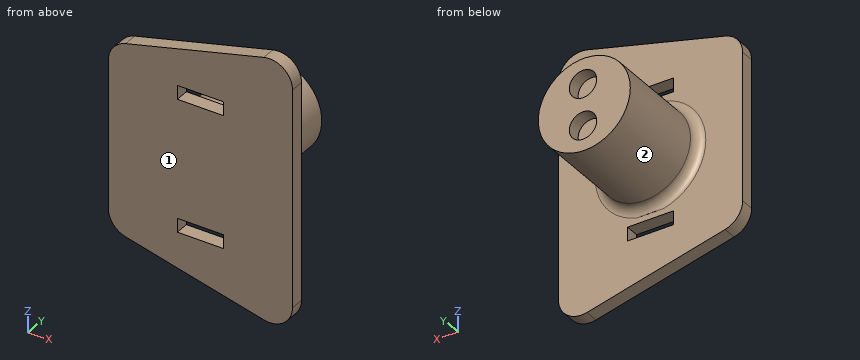
Autodesk Fusion 360 part; units mm, degrees
sketch "Sketch1" plane through (0, 0, 0) normal (0, 1, 0) x (1, 0, 0)
  line L0 (46.0121, 0.2) -> (46.0121, -59.8)
  line L1 (6.0121, -29.5532) -> (6.0121, -9.5532)
  line L2 (6.0121, -29.5532) -> (6.0121, -49.5532)
  line L3 (6.0121, -9.5532) -> (46.0121, 0.2)
  line L4 (6.0121, -49.5532) -> (46.0121, -59.8)
  line L5 (31.0121, -13.6532) -> (21.0121, -13.6532)
  line L6 (21.0121, -13.6532) -> (21.0121, -16.6532)
  line L7 (21.0121, -16.6532) -> (31.0121, -16.6532)
  line L8 (31.0121, -16.6532) -> (31.0121, -13.6532)
  line L9 (31.0121, -42.4532) -> (21.0121, -42.4532)
  line L10 (21.0121, -42.4532) -> (21.0121, -45.4532)
  line L11 (21.0121, -45.4532) -> (31.0121, -45.4532)
  line L12 (31.0121, -45.4532) -> (31.0121, -42.4532)
  point P0 (26.0121, -15.0532)
  point P1 (25.8317, -44.4989)
  dimension "d1" = 60
  dimension "d6" = 20
  dimension "d7" = 20
  dimension "d9" = 40
  dimension "d10" = 40
  dimension "d11" = 20
  dimension "d12" = 14.5
  dimension "d13" = 10
  dimension "d14" = 3
  dimension "d15" = 10
  dimension "d16" = 3
  dimension "d19" = 12.9
  dimension "d20" = 12.9
  dimension "d21" = 25.8
  dimension "d22" = 15
  dimension "d23" = 15
extrude "Extrude1" add sketch "Sketch1" along normal blind 3
sketch "Sketch2" plane through (0, 3, 0) normal (0, 1, 0) x (-1, 0, 0)
  line L0 (-31.0121, 42.4532) -> (-31.0121, 45.4532)
  line L1 (-31.0121, 45.4532) -> (-21.0121, 45.4532)
  line L2 (-21.0121, 45.4532) -> (-21.0121, 42.4532)
  line L3 (-21.0121, 42.4532) -> (-31.0121, 42.4532)
  line L4 (-31.0121, 13.6532) -> (-31.0121, 16.6532)
  line L5 (-31.0121, 16.6532) -> (-21.0121, 16.6532)
  line L6 (-21.0121, 16.6532) -> (-21.0121, 13.6532)
  line L7 (-21.0121, 13.6532) -> (-31.0121, 13.6532)
  line L8 (-6.0121, 9.5532) -> (-6.0121, 49.5532)
  line L9 (-6.0121, 49.5532) -> (-46.0121, 59.8)
  line L10 (-46.0121, 59.8) -> (-46.0121, -0.2)
  line L11 (-46.0121, -0.2) -> (-6.0121, 9.5532)
  circle A0 centre (-26.0121, 29.5532) radius 10
  point P0 (-26.0121, 29.5532)
  dimension "d38" = 12.9
  dimension "d39" = 12.9
  dimension "d42" = 20
extrude "Extrude2" add sketch "Sketch2" along normal blind 22 contours A0
sketch "Sketch3" plane through (0, 25, 0) normal (0, 1, 0) x (-1, 0, 0)
  line L0 (-28.0121, 38.7532) -> (-24.0121, 38.7532)
  line L1 (-24.0121, 38.7532) -> (-24.0121, 20.7532)
  line L2 (-24.0121, 20.7532) -> (-28.0121, 20.7532)
  line L3 (-28.0121, 20.7532) -> (-28.0121, 38.7532)
  line L4 (-28.0121, 38.7532) -> (-24.0121, 20.7532) construction
  line L5 (-24.0121, 38.7532) -> (-28.0121, 20.7532) construction
  circle A0 centre (-26.0121, 29.5532) radius 10
  point P0 (-26.0121, 29.7532)
  dimension "d28" = 18
fillet "Fillet4" radius 2 1 edges at (35.3354, 3, 33.1694)
fillet "Fillet3" radius 5 4 edges at (6.0121, 1.5, 9.5532) (6.0121, 1.5, 49.5532) (46.0121, 1.5, 59.8) (46.0121, 1.5, -0.2)
sketch "Sketch5" plane through (0, 25, 0) normal (0, 1, 0) x (-1, 0, 0)
  circle A0 centre (-26.0121, 29.5532) radius 10
  circle A1 centre (-26.282, 34.0532) radius 2.975
  circle A2 centre (-26.282, 25.0532) radius 2.975
  dimension "d48" = 5.95
  dimension "d49" = 5.95
  dimension "d50" = 4.5
  dimension "d51" = 4.5
extrude "Extrude5" cut sketch "Sketch5" against normal blind 2.93 contours A1 | A2
sketch "Sketch6" plane through (0, 3, 0) normal (0, 1, 0) x (-1, 0, 0)
  arc A0 (-46.0121, 6.1656) -> (-39.8276, 1.308) centre (-41.0121, 6.1656) ccw
  line L0 (-39.8276, 1.308) -> (-9.8276, 8.6229)
  arc A1 (-9.8276, 8.6229) -> (-6.0121, 13.4806) centre (-11.0121, 13.4806) ccw
  line L1 (-6.0121, 13.4806) -> (-6.0121, 45.6726)
  arc A2 (-6.0121, 45.6726) -> (-9.7713, 50.5162) centre (-11.0121, 45.6726) ccw
  line L2 (-9.7713, 50.5162) -> (-39.7713, 58.2013)
  arc A3 (-39.7713, 58.2013) -> (-46.0121, 53.3577) centre (-41.0121, 53.3577) ccw
  line L3 (-46.0121, 53.3577) -> (-46.0121, 6.1656)
  line L4 (-31.0121, 42.4532) -> (-31.0121, 45.4532)
  line L5 (-31.0121, 45.4532) -> (-21.0121, 45.4532)
  line L6 (-21.0121, 45.4532) -> (-21.0121, 42.4532)
  line L7 (-21.0121, 42.4532) -> (-31.0121, 42.4532)
  line L8 (-31.0121, 13.6532) -> (-31.0121, 16.6532)
  line L9 (-31.0121, 16.6532) -> (-21.0121, 16.6532)
  line L10 (-21.0121, 16.6532) -> (-21.0121, 13.6532)
  line L11 (-21.0121, 13.6532) -> (-31.0121, 13.6532)
  circle A4 centre (-26.0121, 29.5532) radius 12
  line L12 (-21.0121, 17.9232) -> (-31.0121, 17.9232)
  line L13 (-31.0121, 17.9232) -> (-31.0121, 12.3832)
  line L14 (-31.0121, 12.3832) -> (-21.0121, 12.3832)
  line L15 (-21.0121, 12.3832) -> (-21.0121, 17.9232)
  line L16 (-21.0121, 17.9232) -> (-31.0121, 12.3832) construction
  line L17 (-31.0121, 17.9232) -> (-21.0121, 12.3832) construction
  line L18 (-31.0121, 41.1832) -> (-21.0121, 41.1832)
  line L19 (-21.0121, 41.1832) -> (-21.0121, 46.7232)
  line L20 (-21.0121, 46.7232) -> (-31.0121, 46.7232)
  line L21 (-31.0121, 46.7232) -> (-31.0121, 41.1832)
  line L22 (-31.0121, 41.1832) -> (-21.0121, 46.7232) construction
  line L23 (-21.0121, 41.1832) -> (-31.0121, 46.7232) construction
  point P0 (-26.0121, 15.1532)
  point P1 (-26.0121, 43.9532)
  dimension "d52" = 10
  dimension "d53" = 5.54
  dimension "d54" = 5.54
extrude "Extrude6" cut sketch "Sketch6" along normal blind 11 contours L7 A4 L18 L19 L21 | A4 L18 | A4 L12 | L9 A4 L12 L13 L15
equation "d12 = ( 29 / 2 ) * 1 mm"
equation "d26 = 37 mm - 10 mm - 5 mm"
The listing builds one solid part. Answer for the finished solid, in the listing's coordinates (mm). Face numbers are marked on the shaded views. A direction names the side the tool comes from. Round coordinates to 2 decimals unless told otherwise and drop trailing zeros. Order: outer loops, then holes, each group sorted by start corner. A loop starts at its lowest first (then second) coordinate and runs counter-clockwise, first axis right, second up. Notation, with made-up numbers: (-8.75, -17.75) - (-4.75, -17.75) arc R17 ccw to (-4.75, 8.25) - close; hole circle Ø8 at (73.25, -38.75). An arc over 180 degrees is marked (long way). Write item = value, one per line. Start each with the question number.
1) For the marked faces 1 and 2, determine the directions among +Z, -Z, +X, -X, +Y, -Y from which every point of the face is accessible in a straight line to the end or side of a thin tool.
2) Given pin 1 (1.5 mm diameter, centred on x = 27, y = 1, fed in from -Z); pin 2 (3.5 mm diameter, centred on x = 26.5, y = 1, fed in from +Z); pin 3 (1 mm diameter, centred on y = 20.5, z = 39, fed in from -X) (3 decimals); pin 4 (7 mm diameter, centred on x = 26.28, z = 25.05, fed in from +Y), each flat-ended and moving along its own axis, determine where each tip first touches the part or whether it passes through.
3) Section B-B, the plane y = 23.25 is taken. Write down the section's boundary in (x, z) (3 decimals), plus the area to 3 significant figures.
4) Section D-D, the plane x = 10.5 is taken. Write down the section's boundary in (y, z), plus the area to 3 significant figures.
5) Straight lines are drawn through the part: L1, parallel to Y at x = 26.5, z = 23.5; L2, parallel to Y at x = 44, z = 49; L3, parallel to Z at x = 26, y = 9. For each, find the intervals that lie inside material, in ascending order.
6) Section C-C, the plane x = 27 is taken. Count the separate pieces of the cut face and the enclosed holes in it, plus the area to 3 significant figures.
7) Section A-A, the plane z = 16 is taken. Write down the section's boundary in (x, y), plus the area to 3 significant figures.
Results list:
q1.face_1 = +Z, -Z, +X, -X, -Y
q1.face_2 = +Y
q2.pin_1 = 4.25
q2.pin_2 = 55.25
q2.pin_3 = 21.545
q2.pin_4 = 25
q3.outline = circle Ø20 at (26.012, 29.553); hole circle Ø5.95 at (26.282, 25.053); hole circle Ø5.95 at (26.282, 34.053)
q3.area = 259 mm^2
q4.outline = (0, 8.46) - (3, 8.46) - (3, 50.7) - (0, 50.7) - close
q4.area = 127 mm^2
q5.L1 = 0 to 22.07
q5.L2 = 0 to 3
q5.L3 = 19.55 to 39.55
q6.separate_pieces = 3
q6.enclosed_holes = 0
q6.area = 539 mm^2
q7.outline = (6.01, 0) - (21.01, 0) - (21.01, 3) - (6.01, 3) - close; (31.01, 0) - (46.01, 0) - (46.01, 3) - (31.01, 3) - close
q7.area = 90.0 mm^2
